from build123d import *

# Parameters (mm, degrees)
HOLE_WIZARD_1_D           = 6.6
HOLE_WIZARD_1_CBORE_D     = 11
HOLE_WIZARD_1_CBORE_DEPTH = 6
CHAMFER_1_SIZE            = 1
CHAMFER_1_SIZE2           = 1.056754503


with BuildPart() as part:
    # 草图1 → 旋转1 (revolve)
    with BuildSketch(Plane.XY):
        Polygon((0, 0), (9, 0), (9, 2), (8.580737766, 10), (0, 10), align=None)
    revolve(axis=Axis((0, -1000, 0), (0, 1, 0)))

    # 打孔尺寸根据内六角圆柱头螺钉的类型1 (through all)
    with Locations(Plane(origin=(0, 10, 0), x_dir=(1, 0, 0), z_dir=(0, 1, 0))):
        with Locations((0, 0)):
            CounterBoreHole(HOLE_WIZARD_1_D / 2, HOLE_WIZARD_1_CBORE_D / 2, HOLE_WIZARD_1_CBORE_DEPTH)

    # 倒角1
    chamfer_1_edges = [part.edges().sort_by_distance(p)[0] for p in [
        (-8.580737766, 10, 0),
    ]]
    chamfer_1_side = [part.faces().sort_by_distance(p)[0] for p in [
        (-8.338037851, 10, 0),
    ]]
    chamfer(chamfer_1_edges, length=CHAMFER_1_SIZE, length2=CHAMFER_1_SIZE2, reference=chamfer_1_side[0])


solid = part.part
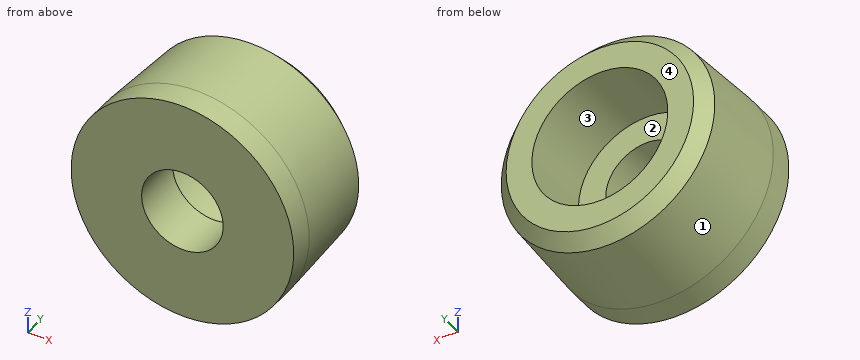
Work out the finished part from the listing and answer in its coordinate system (mm). Face numbers are marked on the shaded views. Round coordinates to 2 decimals unless told otherwise and drop trailing zeros. Loops run counter-clockwise (first coordinate to the right, second up) from the corner with the lowest first, then second, coordinate; pieces in that order, holes last. Notation, with made-up numbers: (-8, 50) - (7, 50) arc R20 cw to (7, 54) - close; hole circle Ø4 at (-24.5, 44). An arc over 180 degrees is marked (long way). One line per item, written item: value.
Q1. Straight lines are drawn through the part: probe 1 along Z at (x, y) = (1.5, 5.5); probe 2 along Z at (x, y) = (0, 6.65); probe 3 along X at (y, z) = (7, 4). For each, find the intervals that lie inside material, in ascending order.
Check values:
probe 1: -8.69 to -5.29, 5.29 to 8.69
probe 2: -8.76 to -5.5, 5.5 to 8.76
probe 3: -7.77 to -3.77, 3.77 to 7.77
Q2. Find section A-A on x = 0. Give the vertices of the cut face in (y, z), and give its area (3 significant figures).
Check values:
outline: (0, -9) - (2, -9) - (8.94, -8.64) - (10, -7.58) - (10, -5.5) - (4, -5.5) - (4, -3.3) - (0, -3.3) - close; (0, 3.3) - (4, 3.3) - (4, 5.5) - (10, 5.5) - (10, 7.58) - (8.94, 8.64) - (2, 9) - (0, 9) - close
area: 83.2 mm2
Q3. Each of these flat-tipped pins is pushed along its axis until it touches: pin 1 Ø4 at (y, z) = (1.5, 2.5) entering from -X; pin 2 Ø1 at (x, y) = (0, 6) entering from -Z; pin 3 Ø5 at (x, y) = (2.5, 5.5) entering from +Z; pin 4 Ø5.5 at (x, z) = (0, 0) entering from +Y. Where does it stop, or does it pass through?
Check values:
pin 1: x = -8.99
pin 2: z = -8.82
pin 3: z = 8.88
pin 4: through
Q4. Find section B-B on z = 0. Give the vertices of the cut face in (x, y).
Check values:
outline: (-9, 0) - (-3.3, 0) - (-3.3, 4) - (-5.5, 4) - (-5.5, 10) - (-7.58, 10) - (-8.64, 8.94) - (-9, 2) - close; (3.3, 0) - (9, 0) - (9, 2) - (8.64, 8.94) - (7.58, 10) - (5.5, 10) - (5.5, 4) - (3.3, 4) - close
Q5. Find section D-D on y = 4.75. Give the vertices of the cut face in (x, z).
Check values:
outline: circle Ø17.71 at (0, 0); hole circle Ø11 at (0, 0)
Q6. The mould has two halves that part along X. Classify the marked faces 1, 2, 3 and 4: +X half, -X half, draft (parallel to the pull), parting line (faces both ways), or undercut.
Check values:
face 1: parting line
face 2: undercut
face 3: undercut
face 4: draft
Q7. Find section C-C on y = 1. Give the vertices of the cut face in (x, z).
Check values:
outline: circle Ø18 at (0, 0); hole circle Ø6.6 at (0, 0)
